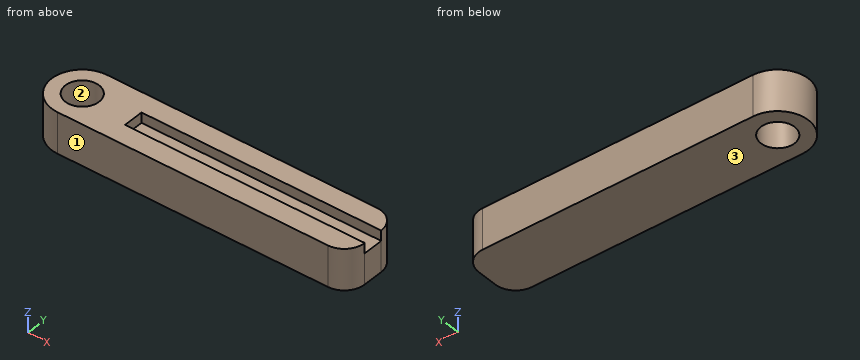
Autodesk Inventor part; units mm, degrees
ref_plane "YZ Plane" through (0, 0, 0) normal (1, 0, 0) x (0, 1, 0)
ref_plane "XZ Plane" through (0, 0, 0) normal (0, 1, 0) x (-1, 0, 0)
ref_plane "XY Plane" through (0, 0, 0) normal (0, 0, 1) x (1, 0, 0)
sketch "Sketch1" plane through (0, 0, 0) normal (0, 0, 1) x (1, 0, 0)
  circle A0 centre (0, 0) radius 1.65
  arc A1 (0, 3) -> (0, -3) centre (0, 0) ccw
  line L0 (0, 3) -> (26.5, 3)
  line L1 (28.5, 1) -> (28.5, -1)
  line L2 (26.5, -3) -> (0, -3)
  arc A2 (28.5, 1) -> (26.5, 3) centre (26.5, 1) ccw
  arc A3 (26.5, -3) -> (28.5, -1) centre (26.5, -1) ccw
  dimension "d0" = 3.3
  dimension "d1" = 6
  dimension "d2" = 2
  dimension "d3" = 28.5
extrude "Extrusion1" add sketch "Sketch1" along normal blind 4
sketch "Sketch2" plane through (0, 0, 4) normal (0, 0, 1) x (1, 0, 0)
  line L0 (52, -1) -> (5, -1)
  line L1 (5, -1) -> (5, 1)
  line L2 (5, 1) -> (52, 1)
  line L3 (52, 1) -> (52, -1)
  line L4 (28.5, -1) -> (28.5, 1)
  line L5 (52, -1) -> (5, 1) construction
  line L6 (5, -1) -> (52, 1) construction
  point P0 (0, 0)
  point P1 (28.5, 0)
  point P2 (28.5, -1)
  point P3 (28.5, 1)
  dimension "d6" = 2
  dimension "d7" = 5
extrude "Extrusion2" cut sketch "Sketch2" against normal blind 1 contours L0 L1 L2 L4
properties part number "espcam-mount"
Geometry: final body of the model. Coordinates: model frame, mm. Face numbers are marked on the shaded views. Give positions to 0.01 mm unless a question says otherwise; leave off trailing zeros. Order: outer loops, then holes, each group sorted by start corner. A loop starts at its lowest first (then second) coordinate and runs counter-clockwise, first axis right, second up. Notation, with made-up numbers: (84.5, -38) -> (113.5, -38) arc R28 ccw to (113.5, 1) -> close; hole circle Ø11 at (17, -15.75). An arc over 180 degrees is marked (long way). Answer as a JSON object with one key per item and string values.
Q1. Draft query along Y for the marked faces 1, 2 and 3. Return one class per face: released by +Y, released by -Y, zero draft, split by the parting line, or undercut.
Entries:
{"face 1": "released by -Y", "face 2": "undercut", "face 3": "zero draft"}
Q2. Section A-A (z = 3.3). Output: boundary loops of the cut face in (x, y), plus the area to 3 significant figures.
Entries:
{"outline": "(0, -3) -> (26.5, -3) arc R2 ccw to (28.5, -1) -> (5, -1) -> (5, 1) -> (28.5, 1) arc R2 ccw to (26.5, 3) -> (0, 3) arc R3 ccw to start; hole circle Ø3.3 at (0, 0)", "area": "128 mm^2"}
Q3. First-contact query: pin 1 (0.8 mm diameter, centred on y = 0, z = 3.5, fed in from +X); pin 2 (0.6 mm diameter, centred on x = 15.5, y = 0, fed in from +Z); pin 3 (1 mm diameter, centred on y = 2, z = 1.5, fed in from -X). Flat tips, straight axial feed; report the tip coordinate or a pass-through.
Entries:
{"pin 1": "stops at x = 5", "pin 2": "stops at z = 3", "pin 3": "stops at x = -2.6"}
Q4. Section D-D (z = 1.2). Output: boundary loops of the cut face in (x, y).
Entries:
{"outline": "(0, -3) -> (26.5, -3) arc R2 ccw to (28.5, -1) -> (28.5, 1) arc R2 ccw to (26.5, 3) -> (0, 3) arc R3 ccw to start; hole circle Ø3.3 at (0, 0)"}
Q5. Section C-C (x = 10). Output: boundary loops of the cut face in (y, z).
Entries:
{"outline": "(-3, 0) -> (3, 0) -> (3, 4) -> (1, 4) -> (1, 3) -> (-1, 3) -> (-1, 4) -> (-3, 4) -> close"}
Q6. Section B-B (y = 0). Output: boundary loops of the cut face in (x, z).
Entries:
{"outline": "(-3, 0) -> (-1.65, 0) -> (-1.65, 4) -> (-3, 4) -> close; (1.65, 0) -> (28.5, 0) -> (28.5, 3) -> (5, 3) -> (5, 4) -> (1.65, 4) -> close"}
Q7. Material intervals for probe 1 along Y at (x, z) = (0, 0.9); probe 2 along Z at (x, y) = (20.5, 0.55); probe 3 along X at (y, z) = (-0.5, 2.45), sorted ascending.
Entries:
{"probe 1": "y = -3 to -1.65, 1.65 to 3", "probe 2": "z = 0 to 3", "probe 3": "x = -2.96 to -1.57, 1.57 to 28.5"}
